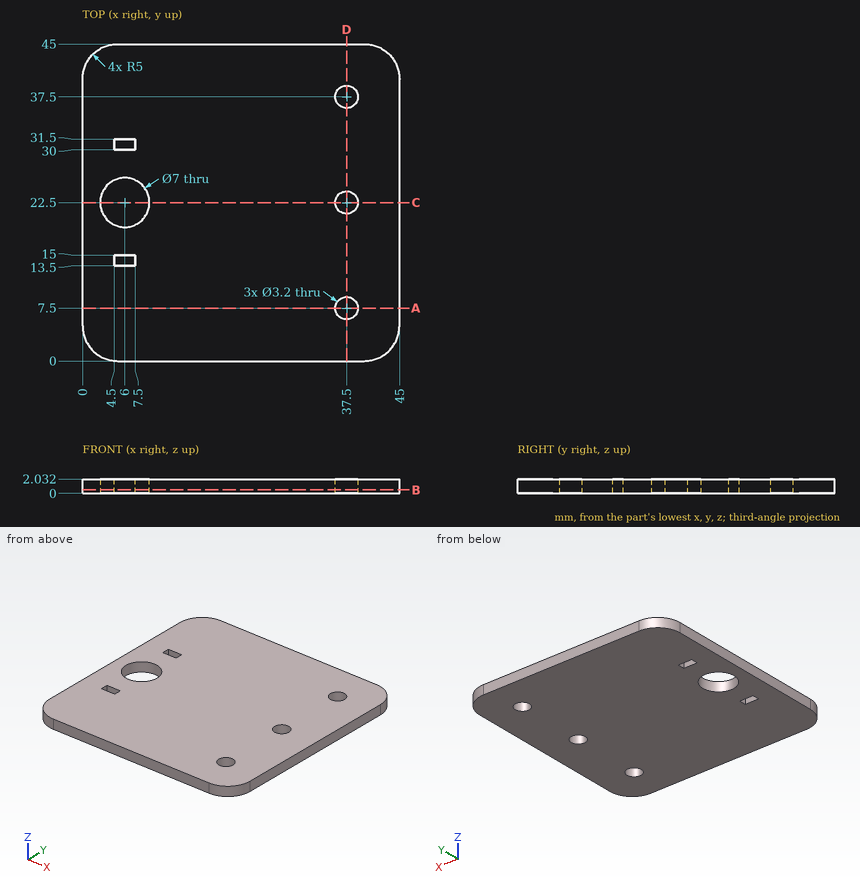
Geometry: see drawing. Coordinates: mm, zero at the bounding-box minimum. Coordinates: 2 decimals unless noted, no trailing zeros. Loops run counter-clockwise (first coordinate to the right, second up) from the corner with the lowest first, then second, coordinate; pieces in that order, holes last. Notation, with made-up numbers: (1.5, 28.25) - (26.5, 28.25) arc R17 ccw to (26.5, 59.25) - close; hole circle Ø1 at (30, 81.5). An arc over 180 degrees is marked (long way). Put each result on its own line as item: value. Start each with the question number.
Q1. Cut plane D-D, the plane x = 37.5. Return loops of the section in (y, z).
Q2. Cut plane B-B, the plane z = 0.5. Return loops of the section in (x, y).
Q3. Cut plane A-A, the plane y = 7.5. Return loops of the section in (x, z), and give its area (3 significant figures).
Q4. Cut plane C-C, the plane y = 22.5. Return loops of the section in (x, z).
Q5. Line query: line 1 (Y direction, x = 6, z = 0.9); line 2 (Y direction, x = 37.5, z = 1.35); line 3 (Y direction, x = 9, z = 0.5). Output: solid intervals per line, ascending.
Filled sheet:
1. outline: (0, 0) - (5.9, 0) - (5.9, 2.03) - (0, 2.03) - close; (9.1, 0) - (20.9, 0) - (20.9, 2.03) - (9.1, 2.03) - close; (24.1, 0) - (35.9, 0) - (35.9, 2.03) - (24.1, 2.03) - close; (39.1, 0) - (45, 0) - (45, 2.03) - (39.1, 2.03) - close
2. outline: (0, 5) arc R5 ccw to (5, 0) - (40, 0) arc R5 ccw to (45, 5) - (45, 40) arc R5 ccw to (40, 45) - (5, 45) arc R5 ccw to (0, 40) - close; hole circle Ø7 at (6, 22.5); hole (4.5, 13.5) - (7.5, 13.5) - (7.5, 15) - (4.5, 15) - close; hole (4.5, 30) - (7.5, 30) - (7.5, 31.5) - (4.5, 31.5) - close; hole circle Ø3.2 at (37.5, 7.5); hole circle Ø3.2 at (37.5, 22.5); hole circle Ø3.2 at (37.5, 37.5)
3. outline: (0, 0) - (35.9, 0) - (35.9, 2.03) - (0, 2.03) - close; (39.1, 0) - (45, 0) - (45, 2.03) - (39.1, 2.03) - close
3. area: 84.9 mm²
4. outline: (0, 0) - (2.5, 0) - (2.5, 2.03) - (0, 2.03) - close; (9.5, 0) - (35.9, 0) - (35.9, 2.03) - (9.5, 2.03) - close; (39.1, 0) - (45, 0) - (45, 2.03) - (39.1, 2.03) - close
5. line 1: 0 to 13.5, 15 to 19, 26 to 30, 31.5 to 45
5. line 2: 0 to 5.9, 9.1 to 20.9, 24.1 to 35.9, 39.1 to 45
5. line 3: 0 to 20.7, 24.3 to 45
